from build123d import *

# Parameters (mm, degrees)
SKETCH1_W           = 30
SKETCH1_H           = 30
BOSS_EXTRUDE1_DEPTH = 10
SKETCH2_W           = 5.5
SKETCH2_H           = 5.5
CUT_EXTRUDE1_DEPTH  = 7.25
FILLET1_R           = 2
SKETCH3_R           = 13.1
CUT_EXTRUDE2_DEPTH  = 7.25
SKETCH4_R           = 1.1
CUT_EXTRUDE3_DEPTH  = 44.041404485
SKETCH5_W           = 22.5
SKETCH5_H           = 8
CUT_EXTRUDE4_DEPTH  = 2
SKETCH6_W           = 2
SKETCH6_H           = 10
CUT_EXTRUDE5_DEPTH  = 1.5
FILLET2_R           = 1
FILLET3_R           = 0.4


# Some blends are built 0.0001 mm under size
with BuildPart() as part:
    # Sketch1 → Boss-Extrude1 (new body)
    with BuildSketch(Plane(origin=(0, 0, 0), x_dir=(1, 0, 0), z_dir=(0, 1, 0))):
        with Locations((15, -15)):
            Rectangle(SKETCH1_W, SKETCH1_H)
    extrude(amount=BOSS_EXTRUDE1_DEPTH)

    # Sketch2 → Cut-Extrude1 (cut)
    with BuildSketch(Plane(origin=(0, 10, 0), x_dir=(1, 0, 0), z_dir=(0, 1, 0))):
        with Locations((27.25, -27.25)):
            Rectangle(SKETCH2_W, SKETCH2_H)
        with Locations((2.75, -2.75)):
            Rectangle(SKETCH2_W, SKETCH2_H)
    extrude(amount=-CUT_EXTRUDE1_DEPTH, mode=Mode.SUBTRACT)

    # Fillet1
    fillet1_edges = [part.edges().sort_by_distance(p)[0] for p in [
        (24.5, 6.375, 24.5),
        (5.5, 6.375, 5.5),
    ]]
    fillet(fillet1_edges, radius=FILLET1_R)

    # Sketch3 → Cut-Extrude2 (cut)
    with BuildSketch(Plane(origin=(0, 10, 0), x_dir=(1, 0, 0), z_dir=(0, 1, 0))):
        with Locations(Location((15.8, -15, 0), (0, 0, 270))):
            Circle(SKETCH3_R)
    extrude(amount=-CUT_EXTRUDE2_DEPTH, mode=Mode.SUBTRACT)

    # Sketch4 → Cut-Extrude3 (cut, through all)
    with BuildSketch(Plane(origin=(0, 2.75, 0), x_dir=(1, 0, 0), z_dir=(0, 1, 0))):
        with Locations(Location((2.75, -2.75, 0), (0, 0, 270))):
            Circle(SKETCH4_R)
        with Locations(Location((27.25, -27.25, 0), (0, 0, 270))):
            Circle(SKETCH4_R)
    extrude(amount=-CUT_EXTRUDE3_DEPTH, mode=Mode.SUBTRACT)

    # Sketch5 → Cut-Extrude4 (cut)
    with BuildSketch(Plane.XY.offset(30)):
        with Locations((12.25, 5)):
            Rectangle(SKETCH5_W, SKETCH5_H)
    extrude(amount=-CUT_EXTRUDE4_DEPTH, mode=Mode.SUBTRACT)

    # Sketch6 → Cut-Extrude5 (cut)
    with BuildSketch(Plane(origin=(30, 0, 0), x_dir=(0, 0, -1), z_dir=(1, 0, 0))):
        with Locations((-21.8, 5)):
            Rectangle(SKETCH6_W, SKETCH6_H)
    extrude(amount=-CUT_EXTRUDE5_DEPTH, mode=Mode.SUBTRACT)

    # Fillet2
    fillet2_edges = [part.edges().sort_by_distance(p)[0] for p in [
        (30, 1.375, 30),
        (0, 1.375, 0),
        (30, 5, 0),
        (0, 5, 30),
    ]]
    fillet(fillet2_edges, radius=FILLET2_R - 0.0001)  # a hair under: the kernel refuses the full size

    # Fillet3
    # the kernel refuses this fillet: 0.4 mm, written as the material it takes off along each edge
    with BuildSketch(Plane(origin=(4.5, 10, 0), x_dir=(0, 0, 1), z_dir=(1, 0, 0)), Plane(origin=(25.5, 10, 30), x_dir=(0, 0, -1), z_dir=(-1, 0, 0)), Plane(origin=(0, 10, 29.0001), x_dir=(1, 0, 0), z_dir=(0, 0, -1))) as fillet3_piece_1:
        with BuildLine():
            CenterArc((FILLET3_R, FILLET3_R), FILLET3_R, 180, 90)
            Line((0, FILLET3_R), (0, 0))
            Line((0, 0), (FILLET3_R, 0))
        make_face()
    extrude(amount=24.5001, mode=Mode.SUBTRACT)
    with BuildSketch(Plane(origin=(0.9999, 0, 0), x_dir=(0, 1, 0), z_dir=(1, 0, 0)), Plane(origin=(29.0001, 0, 30), x_dir=(0, 1, 0), z_dir=(-1, 0, 0)), Plane(origin=(0, 0, 29.0001), x_dir=(0, 1, 0), z_dir=(0, 0, -1))) as fillet3_piece_2:
        with BuildLine():
            CenterArc((FILLET3_R, FILLET3_R), FILLET3_R, 180, 90)
            Line((0, FILLET3_R), (0, 0))
            Line((0, 0), (FILLET3_R, 0))
        make_face()
    extrude(amount=28.0002, mode=Mode.SUBTRACT)
    with BuildSketch(Plane(origin=(30, 0, 21.8), x_dir=(0, 1, 0), z_dir=(0, 0, 1))) as fillet3_piece_3:
        with BuildLine():
            CenterArc((FILLET3_R, FILLET3_R), FILLET3_R, 180, 90)
            Line((0, FILLET3_R), (0, 0))
            Line((0, 0), (FILLET3_R, 0))
        make_face()
    extrude(amount=7.2001, mode=Mode.SUBTRACT)
    with BuildSketch(Plane(origin=(0.9999, 0, 0.9999), x_dir=(-1, 0, 0), z_dir=(0, 0, 1))) as fillet3_piece_4:
        with BuildLine():
            CenterArc((0.9999 - FILLET3_R, -FILLET3_R), FILLET3_R, 0, 90)
            Line((0.9999, -FILLET3_R), (0.9999, 0))
            Line((0.9999, 0), (0.9999 - FILLET3_R, 0))
        make_face()
    revolve(axis=Axis((0.9999, 0, 0.9999), (0, -1, 0)), revolution_arc=90, mode=Mode.SUBTRACT)
    with BuildSketch(Plane(origin=(0.9999, 0, 29.0001), x_dir=(-1, 0, 0), z_dir=(0, 0, -1))) as fillet3_piece_5:
        with BuildLine():
            CenterArc((0.9999 - FILLET3_R, FILLET3_R), FILLET3_R, 270, 90)
            Line((0.9999 - FILLET3_R, 0), (0.9999, 0))
            Line((0.9999, 0), (0.9999, FILLET3_R))
        make_face()
    revolve(axis=Axis((0.9999, 0, 29.0001), (0, 1, 0)), revolution_arc=90, mode=Mode.SUBTRACT)
    with BuildSketch(Plane(origin=(29.0001, 0, 29.0001), x_dir=(0, 0, 1), z_dir=(-1, 0, 0))) as fillet3_piece_6:
        with BuildLine():
            CenterArc((0.9999 - FILLET3_R, FILLET3_R), FILLET3_R, 270, 90)
            Line((0.9999, FILLET3_R), (0.9999, 0))
            Line((0.9999, 0), (0.9999 - FILLET3_R, 0))
        make_face()
    revolve(axis=Axis((29.0001, 0, 29.0001), (0, 1, 0)), revolution_arc=90, mode=Mode.SUBTRACT)
    with BuildSketch(Plane(origin=(29.0001, 0, 0.9999), x_dir=(1, 0, 0), z_dir=(0, 0, 1))) as fillet3_piece_7:
        with BuildLine():
            CenterArc((0.9999 - FILLET3_R, FILLET3_R), FILLET3_R, 270, 90)
            Line((0.9999 - FILLET3_R, 0), (0.9999, 0))
            Line((0.9999, 0), (0.9999, FILLET3_R))
        make_face()
    revolve(axis=Axis((29.0001, 0, 0.9999), (0, 1, 0)), revolution_arc=90, mode=Mode.SUBTRACT)
    with BuildSketch(Plane(origin=(0.9999, 10, 29.0001), x_dir=(-1, 0, 0), z_dir=(0, 0, -1))) as fillet3_piece_8:
        with BuildLine():
            CenterArc((0.9999 - FILLET3_R, -FILLET3_R), FILLET3_R, 0, 90)
            Line((0.9999, -FILLET3_R), (0.9999, 0))
            Line((0.9999, 0), (0.9999 - FILLET3_R, 0))
        make_face()
    revolve(axis=Axis((0.9999, 10, 29.0001), (0, 1, 0)), revolution_arc=90, mode=Mode.SUBTRACT)
    with BuildSketch(Plane(origin=(29.0001, 10, 0.9999), x_dir=(1, 0, 0), z_dir=(0, 0, 1))) as fillet3_piece_9:
        with BuildLine():
            CenterArc((0.9999 - FILLET3_R, -FILLET3_R), FILLET3_R, 0, 90)
            Line((0.9999, -FILLET3_R), (0.9999, 0))
            Line((0.9999, 0), (0.9999 - FILLET3_R, 0))
        make_face()
    revolve(axis=Axis((29.0001, 10, 0.9999), (0, 1, 0)), revolution_arc=90, mode=Mode.SUBTRACT)
    with BuildSketch(Plane(origin=(30, 10, 21.8), x_dir=(-1, 0, 0), z_dir=(0, 0, 1))) as fillet3_piece_10:
        with BuildLine():
            CenterArc((FILLET3_R, FILLET3_R), FILLET3_R, 180, 90)
            Line((0, FILLET3_R), (0, 0))
            Line((0, 0), (FILLET3_R, 0))
        make_face()
    extrude(amount=3.7, mode=Mode.SUBTRACT)
    with BuildSketch(Plane(origin=(26.5, 10, 24.5), x_dir=(0, 0, -1), z_dir=(1, 0, 0)), Plane(origin=(3.5, 10, 5.5), x_dir=(0, 0, 1), z_dir=(-1, 0, 0)), Plane(origin=(5.5, 10, -1), x_dir=(1, 0, 0), z_dir=(0, 0, 1)), Plane(origin=(24.5, 10, 31), x_dir=(-1, 0, 0), z_dir=(0, 0, -1))) as fillet3_piece_11:
        with BuildLine():
            CenterArc((FILLET3_R, -FILLET3_R), FILLET3_R, 90, 90)
            Line((0, -FILLET3_R), (0, 0))
            Line((0, 0), (FILLET3_R, 0))
        make_face()
    extrude(amount=4.5, mode=Mode.SUBTRACT)
    with BuildSketch(Plane(origin=(3.5, 10, 3.5), x_dir=(1, 0, 0), z_dir=(0, 0, -1))) as fillet3_piece_12:
        with BuildLine():
            CenterArc((2 + FILLET3_R, FILLET3_R), FILLET3_R, 180, 90)
            Line((2, FILLET3_R), (2, 0))
            Line((2, 0), (2 + FILLET3_R, 0))
        make_face()
    revolve(axis=Axis((3.5, 10, 3.5), (0, -1, 0)), revolution_arc=90, mode=Mode.SUBTRACT)
    with BuildSketch(Plane(origin=(26.5, 10, 26.5), x_dir=(0, 0, -1), z_dir=(1, 0, 0))) as fillet3_piece_13:
        with BuildLine():
            CenterArc((2 + FILLET3_R, -FILLET3_R), FILLET3_R, 90, 90)
            Line((2, -FILLET3_R), (2, 0))
            Line((2, 0), (2 + FILLET3_R, 0))
        make_face()
    revolve(axis=Axis((26.5, 10, 26.5), (0, 1, 0)), revolution_arc=90, mode=Mode.SUBTRACT)
    with BuildSketch(Plane(origin=(15.8, 10, 15), x_dir=(0, 0, 1), z_dir=(-1, 0, 0))) as fillet3_piece_14:
        with BuildLine():
            CenterArc((13.1 + FILLET3_R, -FILLET3_R), FILLET3_R, 90, 90)
            Line((13.1, -FILLET3_R), (13.1, 0))
            Line((13.1, 0), (13.1 + FILLET3_R, 0))
        make_face()
    revolve(axis=Axis((15.8, 10, 15), (0, 1, 0)), mode=Mode.SUBTRACT)
    with BuildSketch(Plane(origin=(30, 0, 0.9999), x_dir=(0, 1, 0), z_dir=(0, 0, 1)), Plane(origin=(30, 10, 0.9999), x_dir=(-1, 0, 0), z_dir=(0, 0, 1))) as fillet3_piece_15:
        with BuildLine():
            CenterArc((FILLET3_R, FILLET3_R), FILLET3_R, 180, 90)
            Line((0, FILLET3_R), (0, 0))
            Line((0, 0), (FILLET3_R, 0))
        make_face()
    extrude(amount=20.8001, mode=Mode.SUBTRACT)
    with BuildSketch(Plane(origin=(28.5, 10, 20.8), x_dir=(-1, 0, 0), z_dir=(0, 0, 1))) as fillet3_piece_16:
        with BuildLine():
            CenterArc((FILLET3_R, FILLET3_R), FILLET3_R, 180, 90)
            Line((0, FILLET3_R), (0, 0))
            Line((0, 0), (FILLET3_R, 0))
        make_face()
    extrude(amount=2, mode=Mode.SUBTRACT)


solid = part.part
Work out the finished part from the listing and answer in its coordinate system (mm). A direction names the side the tool comes from. Give positions to 0.01 mm unless a question says otherwise; leave off trailing zeros. Loops run counter-clockwise (first coordinate to the right, second up) from the corner with the lowest first, then second, coordinate; pieces in that order, holes last. Notation, with made-up numbers: (53.5, 73.5) -> (98.5, 73.5) arc R24 cw to (98.5, 110.5) -> close; hole circle Ø9 at (56, -6). An arc over 180 degrees is marked (long way). Use a Markdown table: item, result. Add a question column.
1) Each of these flat-tipped pins is pushed along its axis until it touches: P1, Ø1.5, axis at x = 29.5, y = 5.5, coming from the +Z side; P2, Ø1, axis at y = 6.5, z = 29.5, coming from the +X side; P3, Ø3.5, axis at x = 2.75, z = 2.75, coming from the +Y side. Where does it stop, or does it pass through?
2) Which of the six approach directions +Z, -Z, +X, -X, +Y, -Y give full straight-line access (tool end or side, diameter ignored) to faces 1 (the flat face through (2, 6, 5.5)), 2 (the cylindrical face through (10.78, 6.22, 27.1)), 3 (the flat face through (28.5, 5, 22)), 4 (the flat face through (12, 9, 29)), 5 (the flat face through (28, 6, 24.5))?
3) For a pull along Z with two mould halves and no side action, classify faces 6 (the flat face through (1, 5, 29)), 7 (the flat face through (29, 5, 22.8)), 8 (the cylindrical face through (3.08, 1.39, 3.8)), 9 (the cylindrical face through (29.699, 1.591, 29.715)) as +Z half, -Z half, draft (parallel to the pull), parting line (faces both ways), or undercut.
4) Consider line 1 along Y through (x, z) = (21, 28.5); line 2 along X through (y, z) = (1.9, 27.25); line 3 along Y through (x, z) = (26, 16.25). Determine where each line is inside the solid, lowest interval first.
5) The part is cut by section B-B, the plane z = 15. Determine the outline of the cut face in (x, y).
6) The part is cut by section A-A, the plane y = 1.5. Count the separate pieces of the cut face and the enclosed holes in it, plus the area to 3 significant figures.
Reported:
| question | item | result |
|---|---|---|
| 1 | P1 | stops at z = 24.5 |
| 1 | P2 | stops at x = 24.5 |
| 1 | P3 | stops at y = 2.75 |
| 2 | face 1 | -Z, -X, +Y |
| 2 | face 2 | +Y |
| 2 | face 3 | +X, +Y, -Y |
| 2 | face 4 | +Z |
| 2 | face 5 | +Z, +X, +Y |
| 3 | face 6 | draft |
| 3 | face 7 | undercut |
| 3 | face 8 | undercut |
| 3 | face 9 | +Z half |
| 4 | line 1 | y = 0 to 1, 9 to 10 |
| 4 | line 2 | x = 0 to 26.15, 28.35 to 30 |
| 4 | line 3 | y = 0 to 2.75 |
| 5 | outline | (0, 0.4) arc R0.4 ccw to (0.4, 0) -> (29.6, 0) arc R0.4 ccw to (30, 0.4) -> (30, 9.6) arc R0.4 ccw to (29.6, 10) -> (29.3, 10) arc R0.4 ccw to (28.9, 9.6) -> (28.9, 2.75) -> (2.7, 2.75) -> (2.7, 9.6) arc R0.4 ccw to (2.3, 10) -> (0.4, 10) arc R0.4 ccw to (0, 9.6) -> close |
| 6 | separate pieces | 1 |
| 6 | enclosed holes | 2 |
| 6 | area | 844 mm^2 |
